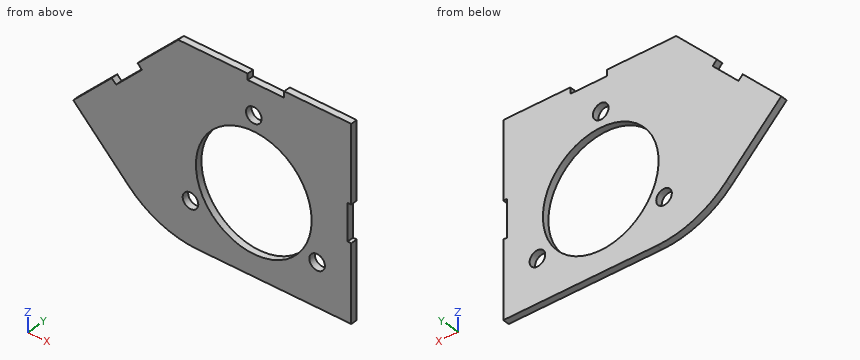
```python
from build123d import *

# Parameters (mm, degrees)
F0_R     = 4.064
F0_R_2   = 30.1625
F1_DEPTH = 3.429


# Not quite as in the source:
# - ends of sketch curves that miss each other by under 0.0002 mm in the source are joined


with BuildPart() as f1:
    # F0 (on Front) → F1 (new body)
    with BuildSketch(Plane.XZ):
        with BuildLine():
            Line((-405.5923562, 237.0029296), (-419.0627382, 223.5325476))
            Line((-419.0627382, 223.5325476), (-421.3077934, 225.7776028))
            Line((-421.3077934, 225.7776028), (-441.368434, 205.7169622))
            Line((-441.368434, 205.7169622), (-412.5468254, 176.895379))
            ThreePointArc((-412.5468254, 176.895379), (-396.0661335641, 165.8833089484), (-376.6258152, 162.0163892))
            Line((-376.6258152, 162.0163892), (-296.474007, 162.0163892))
            Line((-296.474007, 162.0163892), (-296.474007, 201.7038892))
            Line((-296.474007, 201.7038892), (-298.379007, 201.7038892))
            Line((-298.379007, 201.7038892), (-298.379007, 220.7538892))
            Line((-298.379007, 220.7538892), (-296.474007, 220.7538892))
            Line((-296.474007, 220.7538892), (-296.474007, 260.4413892))
            Line((-296.474007, 260.4413892), (-331.399007, 260.4413892))
            Line((-331.399007, 260.4413892), (-331.399007, 257.2663892))
            Line((-331.399007, 257.2663892), (-350.449007, 257.2663892))
            Line((-350.449007, 257.2663892), (-350.449007, 260.4413892))
            Line((-350.449007, 260.4413892), (-386.644007, 260.4413892))
            Line((-386.644007, 260.4413892), (-407.8374114, 239.2479848))
            Line((-407.8374114, 239.2479848), (-405.5923562, 237.0029296))
        make_face()
        with Locations((-380.2695722, 184.2413892)):
            Circle(F0_R, mode=Mode.SUBTRACT)
        with Locations((-314.2784418, 184.2413892)):
            Circle(F0_R, mode=Mode.SUBTRACT)
        with Locations((-347.274007, 203.2913892)):
            Circle(F0_R_2, mode=Mode.SUBTRACT)
        with Locations((-347.274007, 241.3913892)):
            Circle(F0_R, mode=Mode.SUBTRACT)
    extrude(amount=F1_DEPTH)


solid = f1.part
```
Input: part model. Units: mm. Frame: model coordinates. Give positions to 0.01 mm unless a question says otherwise; leave off trailing zeros. Write each loop counter-clockwise with the first axis right and the second up, starting at its lowest first coordinate (ties: lowest second). Pieces come first, ordered by that corner, then holes. Notation, with made-up numbers: (-6.5, 10.25) - (27.5, 10.25) arc R19 cw to (27.5, 40.25) - close; hole circle Ø5 at (41.5, 36). An arc over 180 degrees is marked (long way). Write item = value, one per line. Start each with the question number.
1. Section query D-D, the plane z = 208. Output: boundary loops of the cut face in (x, y), then the cut area to 3 significant figures.
2. Section query A-A, the plane x = -346. Output: boundary loops of the cut face in (y, z).
3. Ray query, L1, parallel to Z at x = -349.5, y = -3.2; L2, parallel to X at y = -3.2, z = 184; L3, parallel to Z at x = -314, y = -0.8. Return the intervals inside material, ascending.
4. First-contact query: pin 1 Ø1 at (x, y) = (-338.5, -1.5) entering from +Z; pin 2 Ø1 at (y, z) = (-2, 258.5) entering from -X; pin 3 Ø2 at (x, y) = (-389.5, -2) entering from -Z. Flat tips, straight axial feed; report the tip coordinate or a pass-through.
5. Section query C-C, the plane y = -0.75. Output: boundary loops of the cut face in (x, z) (1 decimal), then the cut area to 3 significant figures.
6. Section query B-B, the plane z = 244. Output: boundary loops of the cut face in (x, y), then the cut area to 3 significant figures.
Check sheet entries:
q1.outline = (-439.09, -3.43) - (-377.07, -3.43) - (-377.07, 0) - (-439.09, 0) - close; (-317.48, -3.43) - (-298.38, -3.43) - (-298.38, 0) - (-317.48, 0) - close
q1.area = 278 mm2
q2.outline = (-3.43, 162.02) - (0, 162.02) - (0, 173.16) - (-3.43, 173.16) - close; (-3.43, 233.43) - (0, 233.43) - (0, 237.53) - (-3.43, 237.53) - close; (-3.43, 245.25) - (0, 245.25) - (0, 257.27) - (-3.43, 257.27) - close
q3.L1 = 162.02 to 173.21, 233.37 to 237.99, 244.79 to 257.27
q3.L2 = -419.65 to -384.33, -376.21 to -370.46, -324.09 to -318.34, -310.22 to -296.47
q3.L3 = 162.02 to 180.19, 188.3 to 260.44
q4.pin_1 = 257.27
q4.pin_2 = -389.09
q4.pin_3 = 163.42
q5.outline = (-441.4, 205.7) - (-412.5, 176.9) arc R50.8 ccw to (-376.6, 162) - (-296.5, 162) - (-296.5, 201.7) - (-298.4, 201.7) - (-298.4, 220.8) - (-296.5, 220.8) - (-296.5, 260.4) - (-331.4, 260.4) - (-331.4, 257.3) - (-350.4, 257.3) - (-350.4, 260.4) - (-386.6, 260.4) - (-407.8, 239.2) - (-405.6, 237) - (-419.1, 223.5) - (-421.3, 225.8) - close; hole circle Ø8.1 at (-380.3, 184.2); hole circle Ø60.3 at (-347.3, 203.3); hole circle Ø8.1 at (-347.3, 241.4); hole circle Ø8.1 at (-314.3, 184.2)
q5.area = 8,580 mm2
q6.outline = (-403.09, -3.43) - (-350.39, -3.43) - (-350.39, 0) - (-403.09, 0) - close; (-344.16, -3.43) - (-296.47, -3.43) - (-296.47, 0) - (-344.16, 0) - close
q6.area = 344 mm2
